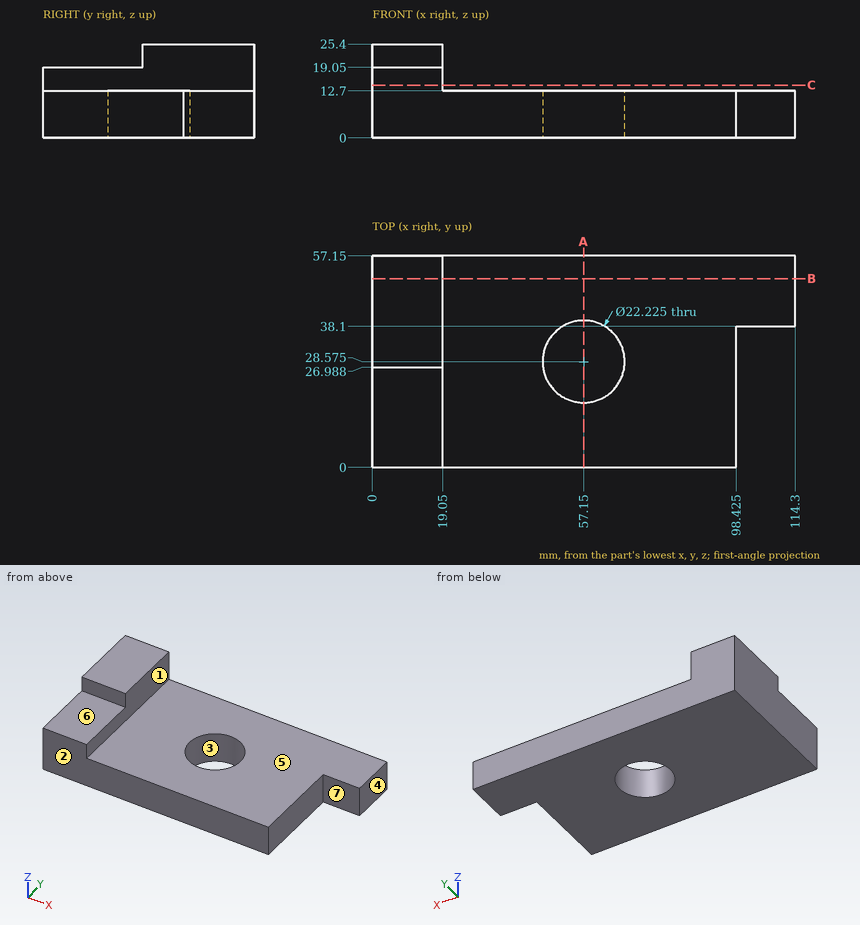
Verification items for this drawing (mm, ordinates from the low corner). A direction names the side the tool comes from. Round coordinates to 2 decimals unless told otherwise and drop trailing zeros. Loops run counter-clockwise (first coordinate to the right, second up) from the corner with the lowest first, then second, coordinate; pieces in that order, holes last. Notation, with made-up numbers: (22, -40) -> (39, -40) arc R32 ccw to (39, -3) -> close; hole circle Ø4 at (-29.5, 31.5). An arc over 180 degrees is marked (long way). Write item = value, one per line. Start each with the question number.
1) Set-up check for the marked faces 4, 5, 6 and 7: record each of +Z, -Z, +X, -X, +Y, -Y from which the full face is reachable in a straight line by a thin tool's end or side.
2) Gauge pin test, flat ends, axial feed: pin 1 Ø9.5 at (x, y) = (10.5, 15) entering from +Z; pin 2 Ø4 at (y, z) = (21, 7.5) entering from +X (1 decimal); pin 3 Ø8 at (y, z) = (24.5, 17.5) entering from +X. Record the tip position at first contact, or that the pin passes through.
3) Sectioned sample at C-C, the plane z = 14.25. Record the cut outline in (x, y), plus the area to 3 significant figures.
4) Thickness scan on probe 1 along Y at (x, z) = (57.15, 3.5); probe 2 along Z at (x, y) = (57, 3.5); probe 3 along X at (y, z) = (36.5, 20.5). Record the ranges inside material, lowest first.
5) Release check for a two-part mould opening along Y. For the marked faces 1, 2 and 3 record: released by +Y, released by -Y, zero draft, split by the parting line, or undercut.
6) Sectioned sample at B-B, the plane y = 51. Record the cut outline in (x, z).
7) Sectioned sample at A-A, the plane x = 57.15. Record the cut outline in (y, z).
Results are:
q1.face_4 = +Z, -Z, +X, +Y, -Y
q1.face_5 = +Z, +X, +Y, -Y
q1.face_6 = +Z, +X, -X, -Y
q1.face_7 = +Z, -Z, +X, -Y
q2.pin_1 = 19.05
q2.pin_2 = 98.4
q2.pin_3 = 19.05
q3.outline = (0, 0) -> (19.05, 0) -> (19.05, 57.15) -> (0, 57.15) -> close
q3.area = 1,090 mm^2
q4.probe_1 = 0 to 17.46, 39.69 to 57.15
q4.probe_2 = 0 to 12.7
q4.probe_3 = 0 to 19.05
q5.face_1 = zero draft
q5.face_2 = released by -Y
q5.face_3 = undercut
q6.outline = (0, 0) -> (114.3, 0) -> (114.3, 12.7) -> (19.05, 12.7) -> (19.05, 25.4) -> (0, 25.4) -> close
q7.outline = (0, 0) -> (17.46, 0) -> (17.46, 12.7) -> (0, 12.7) -> close; (39.69, 0) -> (57.15, 0) -> (57.15, 12.7) -> (39.69, 12.7) -> close
